Study the drawing (mm; zero at the part's minimum x, y, z) and answer. Round coordinates to 2 decimals unless told otherwise and drop trailing zeros. Write each loop counter-clockwise with the first axis right and the second up, starting at its lowest first coordinate (ties: lowest second). Pieces come first, ordered by that corner, then holes. Notation, with made-up numbers: (-8, -6) -> (46, -6) arc R12 cw to (46, 4) -> close; hole circle Ø8 at (79, -26.5). An arc over 180 degrees is marked (long way). Write each question's results on one line, items separated by ' | '. Start each with the question number.
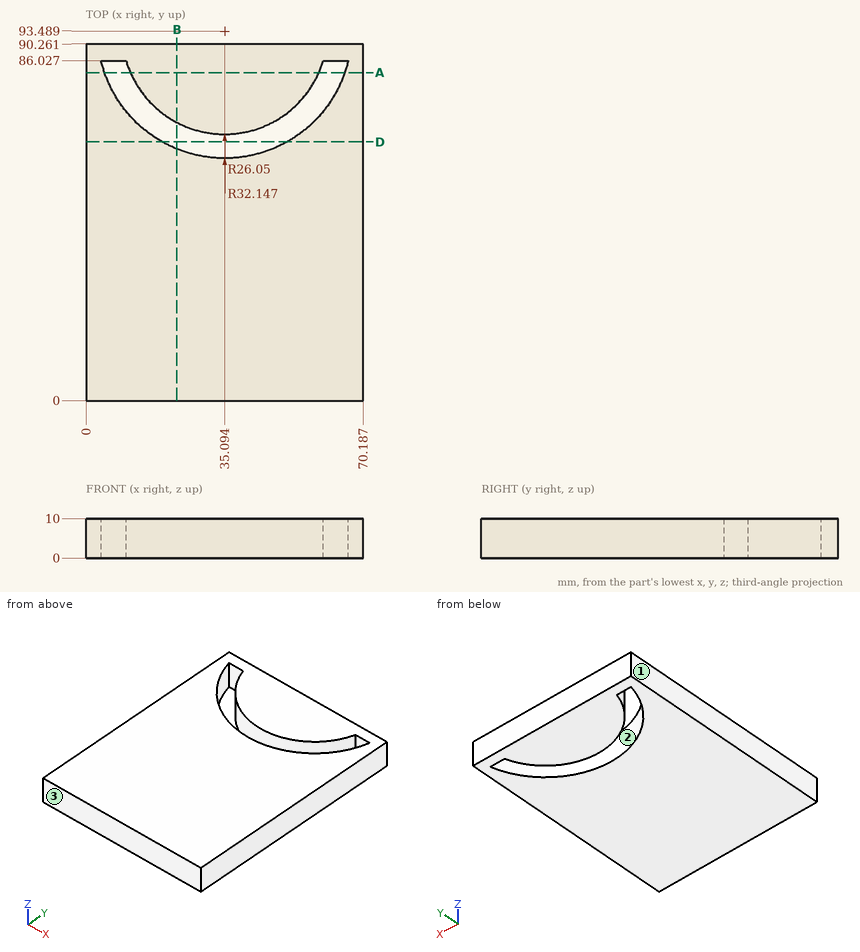
Q1. Find the intervals of material crossed by line 1 (X direction, y = 80.5, z = 1) (1 decimal); line 2 (X direction, y = 85.5, z = 9.5) (1 decimal); line 3 (Y direction, x = 38.5, z = 9), in increasing order.
Q2. The part is cut by section B-B, the plane x = 23. Write down the section's boundary in (y, z).
Q3. The part is cut by section A-A, the plane y = 83. Write down the section's boundary in (x, z) (1 decimal).
Q4. Determine the mould class of the marked faces 1, 2 and 3 for opening direction X: pulls with the +X half, pulls with the -X half, needs draft (parallel to the pull), parting line crosses it, or undercut.
Q5. The part is cut by section D-D, the plane y = 65.5. Write down the section's boundary in (x, z), then the cut area to 3 significant figures.
Answers follow:
1) line 1: 0 to 5.7, 12.5 to 57.7, 64.5 to 70.2 | line 2: 0 to 4, 10.3 to 59.9, 66.2 to 70.2 | line 3: 0 to 61.52, 67.66 to 90.26
2) outline: (0, 0) -> (63.7, 0) -> (63.7, 10) -> (0, 10) -> close; (70.42, 0) -> (90.26, 0) -> (90.26, 10) -> (70.42, 10) -> close
3) outline: (0, 0) -> (4.7, 0) -> (4.7, 10) -> (0, 10) -> close; (11.2, 0) -> (58.9, 0) -> (58.9, 10) -> (11.2, 10) -> close; (65.5, 0) -> (70.2, 0) -> (70.2, 10) -> (65.5, 10) -> close
4) face 1: pulls with the -X half | face 2: undercut | face 3: needs draft
5) outline: (0, 0) -> (19.28, 0) -> (19.28, 10) -> (0, 10) -> close; (50.91, 0) -> (70.19, 0) -> (70.19, 10) -> (50.91, 10) -> close | area: 386 mm^2
